Verification items for the finished model (mm, model axes). Coordinates: 2 decimals unless noted, no trailing zeros. Write each loop counter-clockwise with the first axis right and the second up, starting at its lowest first coordinate (ties: lowest second). Pieces come first, ordered by that corner, then holes. Notation, with made-up numbers: (15, 31.5) -> (41, 31.5) arc R17 ccw to (41, 53.5) -> close; hole circle Ø8 at (83.25, -9). An arc over 180 degrees is marked (long way). Write item = value, one per line. Start each with the question number.
(1) Section check B-B (x = -269.5). Record the cut outline in (y, z), plus the area to 3 significant figures.
(2) Gauge pin test, flat ends, axial feed: pin 1 Ø2.5 at (x, z) = (-277.5, 3.5) entering from -Y; pin 2 Ø4 at (x, z) = (96, 1) entering from -Y. Record the tip position at first contact, or that the pin passes through.
(3) Section check A-A (z = 6). State how many separate pieces and enclosed holes the cut face has, plus the area to 3 significant figures.
(4) Section check C-C (x = -14). Record the cut outline in (y, z).
(5) Material ranges on probe 1 along Y at (x, z) = (-43.5, 1.25); probe 2 along X at (y, z) = (336, 6.5); probe 3 along Y at (x, z) = (-540, 4), recorded low to high. Write a range as [from, to].
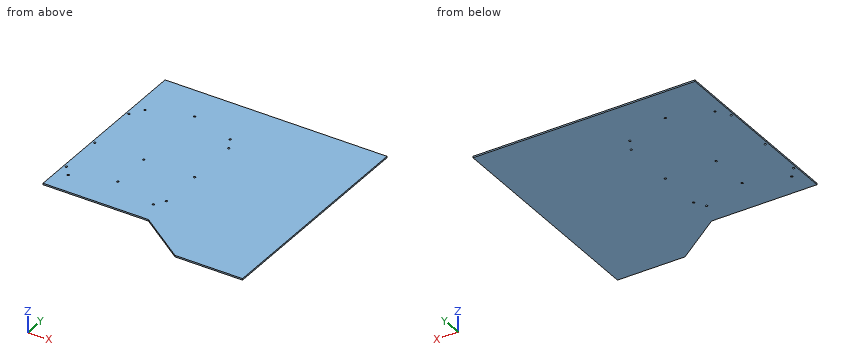
```python
from build123d import *

# Parameters (mm, degrees)
ESTRUSIONE_ESTRUSIONE1_DEPTH = 8
SCHIZZO2_R                   = 5.5
TAGLIO_ESTRUSIONE1_DEPTH     = 8


with BuildPart() as part:
    # Schizzo1 → Estrusione-Estrusione1 (new body)
    with BuildSketch(Plane.XY):
        Polygon((-600, 600), (600, 600), (600, -625), (235, -625), (-30, -435), (-600, -435), align=None)
    extrude(amount=ESTRUSIONE_ESTRUSIONE1_DEPTH)

    # Schizzo2 → Taglio-Estrusione1 (cut)
    with BuildSketch(Plane.XY.offset(8)):
        with Locations((-585, -260)):
            Circle(SCHIZZO2_R)
        with Locations((-540, -315)):
            Circle(SCHIZZO2_R)
        with Locations((-79.872266189, -315)):
            Circle(SCHIZZO2_R)
        with Locations((-44.872266189, -260)):
            Circle(SCHIZZO2_R)
        with Locations((-44.872266189, -20)):
            Circle(SCHIZZO2_R)
        with Locations((-79.872266189, 336)):
            Circle(SCHIZZO2_R)
        with Locations((-540, 336)):
            Circle(SCHIZZO2_R)
        with Locations((-585, -20)):
            Circle(SCHIZZO2_R)
        with Locations((-585, 270)):
            Circle(SCHIZZO2_R)
        with Locations((-44.872266189, 270)):
            Circle(SCHIZZO2_R)
        with Locations((-319.872266189, 411)):
            Circle(SCHIZZO2_R)
        with Locations((-319.872266189, -20)):
            Circle(SCHIZZO2_R)
        with Locations((-319.872266189, -240)):
            Circle(SCHIZZO2_R)
    extrude(amount=-TAGLIO_ESTRUSIONE1_DEPTH, mode=Mode.SUBTRACT)


solid = part.part
```
Response:
q1.outline = (-435, 0) -> (600, 0) -> (600, 8) -> (-435, 8) -> close
q1.area = 8,280 mm2
q2.pin_1 = -435
q2.pin_2 = -526.77
q3.separate_pieces = 1
q3.enclosed_holes = 13
q3.area = 1,340,000 mm2
q4.outline = (-446.47, 0) -> (600, 0) -> (600, 8) -> (-446.47, 8) -> close
q5.probe_1 = [-435, -265.33], [-254.67, -25.33], [-14.67, 264.67], [275.33, 600]
q5.probe_2 = [-600, -545.5], [-534.5, -85.37], [-74.37, 600]
q5.probe_3 = [-435, -320.5], [-309.5, 330.5], [341.5, 600]
